from build123d import *

# Parameters (mm, degrees)
EXTRUDE_1_DEPTH     = 150
CUT_EXTRUDE_1_REACH = 173.828
CUT_EXTRUDE_2_DEPTH = 53
CUT_EXTRUDE_3_DEPTH = 53


with BuildPart() as part:
    # 草图1 → 拉伸1 (new body)
    with BuildSketch(Plane.XY):
        Polygon((0, 40), (0, 50), (5, 50), (25, 40), (25, 0), (5, -30), (0, -30), (0, 0), align=None)
    extrude(amount=EXTRUDE_1_DEPTH)

    # 草图2 → 切除-拉伸1 (cut, up to next)
    with BuildSketch(Plane(origin=(0, 50, 0), x_dir=(-1, 0, 0), z_dir=(0, 1, 0)), mode=Mode.PRIVATE) as cut_extrude_1_sk1:
        Polygon((0, 13.3), (-66.261919137, -14.146585575), (0, -14.146585575), align=None)
    cut_extrude_1_tool1 = extrude(cut_extrude_1_sk1.sketch, amount=-CUT_EXTRUDE_1_REACH, mode=Mode.PRIVATE) & part.part
    # 草图2 → 切除-拉伸1 (cut, up to next)
    with BuildSketch(Plane(origin=(0, 50, 0), x_dir=(-1, 0, 0), z_dir=(0, 1, 0)), mode=Mode.PRIVATE) as cut_extrude_1_sk2:
        Polygon((0, 136.7), (-66.261919137, 164.146585575), (0, 164.146585575), align=None)
    cut_extrude_1_tool2 = extrude(cut_extrude_1_sk2.sketch, amount=-CUT_EXTRUDE_1_REACH, mode=Mode.PRIVATE) & part.part
    add(cut_extrude_1_tool1.solids().sort_by_distance((22.087306, 50, -4.997724))[0], mode=Mode.SUBTRACT)
    add(cut_extrude_1_tool2.solids().sort_by_distance((22.087306, 50, 154.997724))[0], mode=Mode.SUBTRACT)

    # 草图4 → 切除-拉伸2 (cut)
    with BuildSketch(Plane(origin=(0, 0, 18.3), x_dir=(-1, 0, 0), z_dir=(0, 0, -1))):
        Polygon((0, 45), (-6.05572809, 45), (-21, 37.527864045), (-21, 1.211102551), (-3.525931633, -25), (0, -25), align=None)
    extrude(amount=-CUT_EXTRUDE_2_DEPTH, mode=Mode.SUBTRACT)

    # 草图5 → 切除-拉伸3 (cut)
    with BuildSketch(Plane(origin=(0, 0, 131.7), x_dir=(-1, 0, 0), z_dir=(0, 0, -1))):
        Polygon((0, 45), (-6.05572809, 45), (-21, 37.527864045), (-21, 1.211102551), (-3.525931633, -25), (0, -25), align=None)
    extrude(amount=CUT_EXTRUDE_3_DEPTH, mode=Mode.SUBTRACT)


solid = part.part
Could you check a few things on this model? Use its own coordinates, in mm. A direction names the side the tool comes from. Coordinates: 2 decimals unless noted, no trailing zeros. Loops run counter-clockwise (first coordinate to the right, second up) from the corner with the lowest first, then second, coordinate; pieces in that order, holes last.
1. Imagine slicing it at B-B (z = 111). Please give me the cut outline in (x, y), and give its area (3 significant figures).
2. Imagine slicing it at C-C (y = 30.5). Please give me the cut outline in (x, z), and give its area (3 significant figures).
3. I need wall thicknesses on L1, parallel to Y at x = 2.25, z = 101; L2, parallel to Z at x = 4, y = -16.5; L3, parallel to Z at x = 2, y = 24.5. Which ranges of each line are inside material? Lowest first, please.
4. Imagine slicing it at D-D (x = 1.5). Please give me the cut outline in (y, z).
5. For P1, Ø5, axis at y = 17.5, z = 102.5, coming from the -X side; P2, Ø8, axis at x = 19.5, z = 94.5, coming from the -Y side; P3, Ø10.5, axis at x = 10.5, y = 1.5, coming from the +Z side, each with a flat end and sliding along its axis, tell me the tip position at first contact or that it passes through.
6. We'd pull the mould along Z, two halves only. Please class faces 1 (the face through (0, 10, 75)), 2 (the face through (9.547, 10.56, 140.655)), 3 (the face through (21, 20, 106)): released by +Z, released by -Z, zero draft, split by the parting line, or undercut.
7. Imagine slicing it at A-A (x = 14). Please give me the cut outline in (y, z), and give its area (3 significant figures).
8. For faces 4 (the face through (2, 50, 74)), 5 (the face through (13.42, 41.32, 105.57)), which set-ups out of +Z, -Z, +X, -X, +Y, -Y let a thin tool reach every point of the face, with its end or its side?
Computed values:
1. outline: (0, -30) - (5, -30) - (25, 0) - (25, 40) - (5, 50) - (0, 50) - (0, 45) - (6.06, 45) - (21, 37.53) - (21, 1.21) - (3.53, -25) - (0, -25) - close
1. area: 415 mm2
2. outline: (0, 13.3) - (25, 2.94) - (25, 147.06) - (0, 136.7) - (0, 131.7) - (21, 131.7) - (21, 78.7) - (0, 78.7) - (0, 71.3) - (21, 71.3) - (21, 18.3) - (0, 18.3) - close
2. area: 1,120 mm2
3. L1: y = -30 to -25, 45 to 50
3. L2: z = 11.64 to 18.3, 71.3 to 78.7, 131.7 to 138.36
3. L3: z = 12.47 to 18.3, 71.3 to 78.7, 131.7 to 137.53
4. outline: (-30, 12.68) - (50, 12.68) - (50, 137.32) - (-30, 137.32) - close; hole (-25, 18.3) - (45, 18.3) - (45, 71.3) - (-25, 71.3) - close; hole (-25, 78.7) - (45, 78.7) - (45, 131.7) - (-25, 131.7) - close
5. P1: stops at x = 21
5. P2: stops at y = -14.25
5. P3: stops at z = 143.22
6. face 1: zero draft
6. face 2: released by +Z
6. face 3: undercut
7. outline: (-16.5, 7.5) - (45.5, 7.5) - (45.5, 142.5) - (-16.5, 142.5) - close; hole (-9.29, 18.3) - (41.03, 18.3) - (41.03, 71.3) - (-9.29, 71.3) - close; hole (-9.29, 78.7) - (41.03, 78.7) - (41.03, 131.7) - (-9.29, 131.7) - close
7. area: 3,040 mm2
8. face 4: +Z, -Z, +X, -X, +Y
8. face 5: -X
